```python
from build123d import *

# Parameters (mm, degrees)
SKETCH_1_W                  = 24
SKETCH_1_H                  = 36.25
EXTRUDE_1_DEPTH             = 8
CUT_EXTRUDE_1_DEPTH         = 9
HOLE_WIZARD_M31_D           = 2.5
HOLE_WIZARD_M31_DEPTH       = 10.5
HOLE_WIZARD_M31_CSINK_D     = 3.2
HOLE_WIZARD_M31_CSINK_ANGLE = 110
HOLE_WIZARD_M31_TIP         = 0.751075774
HOLE_WIZARD_M33_D           = 2.5
HOLE_WIZARD_M33_DEPTH       = 7
HOLE_WIZARD_M33_CSINK_D     = 3.5
HOLE_WIZARD_M33_CSINK_ANGLE = 110
HOLE_WIZARD_M33_TIP         = 0.751075774
CUT_EXTRUDE_4_DEPTH         = 5


with BuildPart() as part:
    # Эскиз1 → Бобышка-Вытянуть1 (new body)
    with BuildSketch(Plane.XY):
        with Locations((12, 18.125)):
            Rectangle(SKETCH_1_W, SKETCH_1_H)
    extrude(amount=EXTRUDE_1_DEPTH)

    # Эскиз2 → Вырез-Вытянуть1 (cut, through all)
    with BuildSketch(Plane.XY.offset(8)):
        Polygon((-87.021101005, 21.25), (0, 21.25), (3, 21.25), (3, 26.25), (11, 26.25), (11, 0), (11, -87.021101005), (-118.022033053, -203.828648138), (-216.043134058, -95.557547133), align=None)
    extrude(amount=-CUT_EXTRUDE_1_DEPTH, mode=Mode.SUBTRACT)

    # Отверстие обработанное метчиком M31
    with Locations(Plane.XZ):
        with Locations((15, 4), (20, 4)):
            CounterSinkHole(HOLE_WIZARD_M31_D / 2, HOLE_WIZARD_M31_CSINK_D / 2, depth=HOLE_WIZARD_M31_DEPTH, counter_sink_angle=HOLE_WIZARD_M31_CSINK_ANGLE)
            with Locations((0, 0, -(HOLE_WIZARD_M31_DEPTH + HOLE_WIZARD_M31_TIP / 2))):  # 118° drill point
                Cone(0, HOLE_WIZARD_M31_D / 2, HOLE_WIZARD_M31_TIP, mode=Mode.SUBTRACT)

    # Эскиз6 → Отверстие обработанное метчиком M32 (revolve, cut)
    with BuildSketch(Plane(origin=(0, 29.25, 4), x_dir=(0, 0, 1), z_dir=(0, 1, 0))):
        Polygon((0, 0), (0, 24), (1.75, 24), (1.25, 23.649896231), (1.25, 0.350103769), (1.75, 0), align=None)
    revolve(axis=Axis((-6.35, 29.25, 4), (1, 0, 0)), mode=Mode.SUBTRACT)

    # Отверстие обработанное метчиком M33
    with Locations(Plane(origin=(0, 36.25, 0), x_dir=(-1, 0, 0), z_dir=(0, 1, 0))):
        with Locations((-14, 4), (-4, 4), (-21, 4)):
            CounterSinkHole(HOLE_WIZARD_M33_D / 2, HOLE_WIZARD_M33_CSINK_D / 2, depth=HOLE_WIZARD_M33_DEPTH, counter_sink_angle=HOLE_WIZARD_M33_CSINK_ANGLE)
            with Locations((0, 0, -(HOLE_WIZARD_M33_DEPTH + HOLE_WIZARD_M33_TIP / 2))):  # 118° drill point
                Cone(0, HOLE_WIZARD_M33_D / 2, HOLE_WIZARD_M33_TIP, mode=Mode.SUBTRACT)

    # Эскиз11 → Вырез-Вытянуть4 (cut)
    with BuildSketch(Plane(origin=(0, 0, 0), x_dir=(-1, 0, 0), z_dir=(0, 0, -1))):
        with BuildLine():
            ThreePointArc((-10.5, 26.25), (-13.118033989, 26.486067977), (-14.5, 24.25))
            Line((-14.5, 24.25), (-14.5, 23.25))
            ThreePointArc((-14.5, 23.25), (-13.767766953, 21.482233047), (-12, 20.75))
            Line((-12, 20.75), (-12, 0))
            Line((-12, 0), (-11, 0))
            Line((-11, 0), (-11, 26.25))
            Line((-11, 26.25), (-10.5, 26.25))
        make_face()
        Polygon((-0.459002775, 23.25), (-3, 25.029225411), (-3, 21.25), (0, 21.25), (0, 23.25), align=None)
    extrude(amount=-CUT_EXTRUDE_4_DEPTH, mode=Mode.SUBTRACT)


solid = part.part
```
The model under review builds one solid part; all positions refer to its coordinate system, in mm. A direction names the side the tool comes from. Round coordinates to 2 decimals unless told otherwise and drop trailing zeros. Order: outer loops, then holes, each group sorted by start corner. A loop starts at its lowest first (then second) coordinate and runs counter-clockwise, first axis right, second up.
Item 1: For pin 1 (1.5 mm diameter, centred on x = 15, z = 4, fed in from -Y); pin 2 (3 mm diameter, centred on y = 12.5, z = 1, fed in from -X); pin 3 (3 mm diameter, centred on y = 29.25, z = 4, fed in from -X), all flat-tipped, find the tip position at first contact; note any pin that passes through.
Working result:
pin 1: stops at y = 10.8
pin 2: stops at x = 12
pin 3: stops at x = 0.18
Item 2: To check wall thickness, follow probe 1 along X at (y, z) = (31.75, 4); probe 2 along Z at (x, y) = (15, 6); probe 3 along Y at (x, z) = (19.5, 5). State the ranges of each line that lie inside material, in increasing order.
Working result:
probe 1: x = 0 to 2.75, 5.25 to 12.75, 15.25 to 19.75, 22.25 to 24
probe 2: z = 0 to 2.75, 5.25 to 8
probe 3: y = 10.58 to 28.5, 30 to 36.25
Item 3: Draft analysis for pull direction Y (two halves, no side actions). For faces 6 (the cylindrical face through (13.787, 21.502, 2.465)), 7 (the flat face through (14.5, 24, 2)), 8 (the cylindrical face through (18.845, 5.444, 3.521)), 9 (the conical face through (15.12, 11.12, 4.18)), state which applies: released by +Y, released by -Y, zero draft, split by the parting line, or undercut.
Working result:
face 6: undercut
face 7: undercut
face 8: zero draft
face 9: released by -Y
Item 4: Add section A-A, the plane x = 8.5. State the section outline as (y, z) points.
Working result:
outline: (26.25, 0) - (36.25, 0) - (36.25, 8) - (26.25, 8) - close; hole circle Ø2.5 at (29.25, 4)
Item 5: Machinability: for faces 1 (the flat face through (2, 21.25, 7)), 2 (the flat face through (3, 24, 6)), 3 (the cylindrical face through (19.75, 33.27, 4.05)), 4 (the flat face through (14, 22, 8)), 5 (the flat face through (12, 11, 2)), which of the approach directions +Z, -Z, +X, -X, +Y, -Y give a long, thin tool a straight path to every point of the face, cutting with its end or side? Answer none if there is none.
Working result:
face 1: +Z, -Z, -X, -Y
face 2: +Z, -Z, -Y
face 3: +Y
face 4: +Z, +X, -X, +Y, -Y
face 5: -Z, -X, -Y
Item 6: Add section C-C, the plane z = 7. State the section outline as (x, y) points.
Working result:
outline: (0, 21.25) - (3, 21.25) - (3, 26.25) - (11, 26.25) - (11, 0) - (24, 0) - (24, 36.25) - (0, 36.25) - close
Item 7: Add section B-B, the plane y = 3.5. State the section outline as (x, z) points, and give its area (3 significant figures).
Working result:
outline: (11, 5) - (12, 5) - (12, 0) - (24, 0) - (24, 8) - (11, 8) - close; hole circle Ø2.5 at (15, 4); hole circle Ø2.5 at (20, 4)
area: 89.2 mm2
Item 8: Add section D-D, the plane y = 32. State the section outline as (x, z) points, and give its area (3 significant figures).
Working result:
outline: (0, 0) - (24, 0) - (24, 8) - (0, 8) - close; hole circle Ø2.5 at (4, 4); hole circle Ø2.5 at (14, 4); hole circle Ø2.5 at (21, 4)
area: 177 mm2
